```python
from build123d import *

# Parameters (mm, degrees)
SKETCH3_R           = 4
CUT_EXTRUDE1_DEPTH  = 10
SKETCH4_R           = 8
SKETCH4_R_2         = 6.5
BOSS_EXTRUDE1_DEPTH = 4


with BuildPart() as part:
    # Sketch1 → Revolve1 (revolve)
    with BuildSketch(Plane.XY, mode=Mode.PRIVATE) as revolve1_sk:
        Polygon((0, 0), (39, 0), (39, -9), (49, -9), (49, -27.5), (59, -27.5), (59, -31.5), (63, -31.5), (63, -9), (53, -9), (53, 1.623676176), (45, 1.623676176), (45, 29), (40, 29), (40, 5), (0, 5), align=None)
    revolve(revolve1_sk.sketch.rotate(Axis((0, -70, 0), (1, 0, 0)), 90), axis=Axis((0, -70, 0), (1, 0, 0)))

    # Sketch3 → Cut-Extrude1 (cut)
    with BuildSketch(Plane(origin=(45, 0, 0), x_dir=(0, 0, -1), z_dir=(1, 0, 0))):
        with Locations((0, 20)):
            Circle(SKETCH3_R)
        with Locations((77.942286341, -25)):
            Circle(SKETCH3_R)
        with Locations((77.942286341, -115)):
            Circle(SKETCH3_R)
        with Locations((0, -160)):
            Circle(SKETCH3_R)
        with Locations((-77.942286341, -115)):
            Circle(SKETCH3_R)
        with Locations((-77.942286341, -25)):
            Circle(SKETCH3_R)
    extrude(amount=-CUT_EXTRUDE1_DEPTH, mode=Mode.SUBTRACT)

    # Sketch4 → Boss-Extrude1 (add)
    # profile 1 of 6: a face of its own
    with BuildSketch(Plane(origin=(45, 0, 0), x_dir=(0, 0, -1), z_dir=(1, 0, 0))):
        with Locations(Location((0, 20, 0), (0, 0, 180))):
            Circle(SKETCH4_R)
        with Locations((0, 20)):
            Circle(SKETCH4_R_2, mode=Mode.SUBTRACT)
    # profile 2 of 6: a face of its own
    with BuildSketch(Plane(origin=(45, 0, 0), x_dir=(0, 0, -1), z_dir=(1, 0, 0))):
        with Locations(Location((77.942286341, -25, 0), (0, 0, 180))):
            Circle(SKETCH4_R)
        with Locations((77.942286341, -25)):
            Circle(SKETCH4_R_2, mode=Mode.SUBTRACT)
    # profile 3 of 6: a face of its own
    with BuildSketch(Plane(origin=(45, 0, 0), x_dir=(0, 0, -1), z_dir=(1, 0, 0))):
        with Locations(Location((77.942286341, -115, 0), (0, 0, 180))):
            Circle(SKETCH4_R)
        with Locations((77.942286341, -115)):
            Circle(SKETCH4_R_2, mode=Mode.SUBTRACT)
    # profile 4 of 6: a face of its own
    with BuildSketch(Plane(origin=(45, 0, 0), x_dir=(0, 0, -1), z_dir=(1, 0, 0))):
        with Locations(Location((0, -160, 0), (0, 0, 180))):
            Circle(SKETCH4_R)
        with Locations((0, -160)):
            Circle(SKETCH4_R_2, mode=Mode.SUBTRACT)
    # profile 5 of 6: a face of its own
    with BuildSketch(Plane(origin=(45, 0, 0), x_dir=(0, 0, -1), z_dir=(1, 0, 0))):
        with Locations(Location((-77.942286341, -115, 0), (0, 0, 180))):
            Circle(SKETCH4_R)
        with Locations((-77.942286341, -115)):
            Circle(SKETCH4_R_2, mode=Mode.SUBTRACT)
    # profile 6 of 6: a face of its own
    with BuildSketch(Plane(origin=(45, 0, 0), x_dir=(0, 0, -1), z_dir=(1, 0, 0))):
        with Locations(Location((-77.942286341, -25, 0), (0, 0, 180))):
            Circle(SKETCH4_R)
        with Locations((-77.942286341, -25)):
            Circle(SKETCH4_R_2, mode=Mode.SUBTRACT)
    extrude(amount=BOSS_EXTRUDE1_DEPTH)


solid = part.part
```
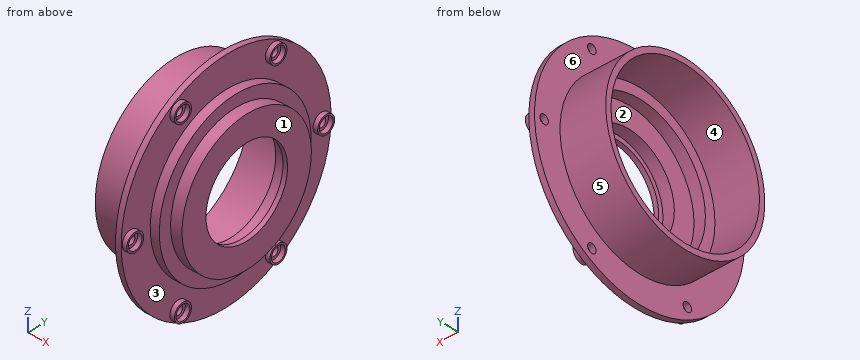
Can you work these out from the model? Positions are in its coordinate system, mm. Face numbers are marked on the shaded views. A direction names the side the tool comes from. Round coordinates to 2 decimals unless told otherwise and drop trailing zeros. Loops run counter-clockwise (first coordinate to the right, second up) from the corner with the lowest first, then second, coordinate; pieces in that order, holes last. Notation, with made-up numbers: M 39,-28 L 70,-28 A21 cw 70,-8 Z; hole C 63.5,-14 d6. An arc over 180 degrees is marked long. Write item = value, one per line. Start each with the question number.
(1) Suppose I cut it at C-C on y = 20. Write out the boundary of the cut face in (x, z), plus the area to 3 significant figures.
(2) I need wall thicknesses on line 1 along Y through (x, z) = (61.25, 0); line 2 along Y through (x, z) = (37.5, 0); line 3 along X through (y, z) = (-18.5, 31). Which ranges of each line are inside material? Lowest first, please.
(3) Which directions (+Z, -Z, +X, -X, +Y, -Y) give clear straight access to the entire face, cutting with the end or side of a thin tool? Please do the marked faces 1, 2 and 3.
(4) I'm going to push flat-ended pins straight in: P1, Ø5, axis at y = 0.5, z = 62, coming from the -X side; P2, Ø5, axis at y = -26.5, z = -79, coming from the +X side; P3, Ø1.5, axis at x = 36.5, z = -35, coming from the -Y side; P4, Ø3, axis at y = -24, z = 51.5, coming from the -X side. Where does each tip first touch, or does it pass through?
(5) Suppose I cut it at D-D on x = 23.5. Write out the boundary of the cut face in (y, z).
(6) If we mould it in two halves opening along Y, with no side actions, what happens to the marked faces 4, 5 and 6? For each: released by +Y, released by -Y, zero draft, split by the parting line, or undercut.
Answer block:
q1.outline = M 40,-41.24 L 45,-41.24 L 45,-8 L 49,-8 L 49,-6.5 L 45,-6.5 L 45,-4 L 40,-4 Z; M 40,4 L 45,4 L 45,6.5 L 49,6.5 L 49,8 L 45,8 L 45,41.24 L 40,41.24 Z
q1.area = 384 mm²
q2.line_1 = -131 to -108.5, -31.5 to -9
q2.line_2 = -145 to -140, 0 to 5
q2.line_3 = 49 to 63
q3.face_1 = +Z, -Z, +X, +Y, -Y
q3.face_2 = -X
q3.face_3 = +X
q4.P1 = 40
q4.P2 = 45
q4.P3 = -136.72
q4.P4 = 0
q5.outline = C -70,0 d150; hole C -70,0 d140
q6.face_4 = undercut
q6.face_5 = split by the parting line
q6.face_6 = zero draft
